For this review, take the finished solid that the model builds, in its own axes (mm). A direction names the side the tool comes from. Round coordinates to 2 decimals unless told otherwise and drop trailing zeros. Write each loop counter-clockwise with the first axis right and the second up, starting at its lowest first coordinate (ties: lowest second). Pieces come first, ordered by that corner, then holes. Notation, with made-up numbers: (2.5, 14.25) -> (7.5, 14.25) arc R28 ccw to (7.5, 34.25) -> close; hole circle Ø8 at (83.25, 35.25). An arc over 180 degrees is marked (long way). Write each question's results on one line, items separated by ' | '. Start each with the question number.
Item 1: Add section B-B (z = 3.7). State the section outline as (x, y) points, plus the area to 3 significant figures.
Item 2: Clearance check with flat-ended pins moving along their axes: pin 1 (1.5 mm diameter, centred on y = 1, z = 2, fed in from +X); pin 2 (3 mm diameter, centred on x = 4, z = 1.5, fed in from -Y); pin 3 (1.5 mm diameter, centred on y = 2.5, z = 2, fed in from +X). State where each tip first meets the part, or that it passes through.
Item 3: To check wall thickness, follow line 1 along Z through (x, y) = (2, -4.75); line 2 along X through (y, z) = (-5.5, 0.55); line 3 along X through (y, z) = (-3.5, 2.7). State the ranges of each line that lie inside material, in increasing order.
Item 4: Add section C-C (z = 0.35). State the section outline as (x, y) points, plus the area to 3 significant figures.
Item 5: Tool access review of faces 1 (the flat face through (0, 0, 5)), 2 (the flat face through (-1.42, -3.92, 2)): name each direction out of +Z, -Z, +X, -X, +Y, -Y from which nothing blocks a thin tool from reaching the whole face with its end or side.
Item 6: Add section A-A (x = 0). State the section outline as (y, z) points, plus the area to 3 significant figures.
from build123d import *

# Parameters (mm, degrees)
F0_R     = 6
F1_DEPTH = 2
F2_R     = 4
F3_DEPTH = 5
F4_R     = 0.5


with BuildPart() as f1:
    # F0 (on Top) → F1 (new body)
    with BuildSketch(Plane.XY):
        Circle(F0_R)
    extrude(amount=F1_DEPTH)

    # F2 (on Top) → F3 (join)
    with BuildSketch(Plane.XY):
        Circle(F2_R)
    extrude(amount=F3_DEPTH)

    # F4
    f4_edges = [f1.edges().sort_by_distance(p)[0] for p in [
        (-6, 0, 0),
    ]]
    fillet(f4_edges, radius=F4_R)


solid = f1.part
Responses:
1) outline: circle Ø8 at (0, 0) | area: 50.3 mm^2
2) pin 1: stops at x = 5.99 | pin 2: stops at y = -5.45 | pin 3: stops at x = 5.74
3) line 1: z = 0 to 2 | line 2: x = -2.4 to 2.4 | line 3: x = -1.94 to 1.94
4) outline: circle Ø11.95 at (0, 0) | area: 112 mm^2
5) face 1: +Z, +X, -X, +Y, -Y | face 2: +Z
6) outline: (-6, 0.5) arc R0.5 ccw to (-5.5, 0) -> (5.5, 0) arc R0.5 ccw to (6, 0.5) -> (6, 2) -> (4, 2) -> (4, 5) -> (-4, 5) -> (-4, 2) -> (-6, 2) -> close | area: 47.9 mm^2
